Study the drawing (mm; zero at the part's minimum x, y, z) and answer. Coordinates: 2 decimals unless noted, no trailing zeros. Loops run counter-clockwise (first coordinate to the right, second up) from the corner with the lowest first, then second, coordinate; pieces in that order, holes last. Notation, with made-up numbers: (20, 15) - (47, 15) arc R8 ccw to (47, 26) - close; hole circle Ø3 at (33, 53). An arc over 180 degrees is marked (long way). Use CSV: the item, a comma, the result in double quotes.
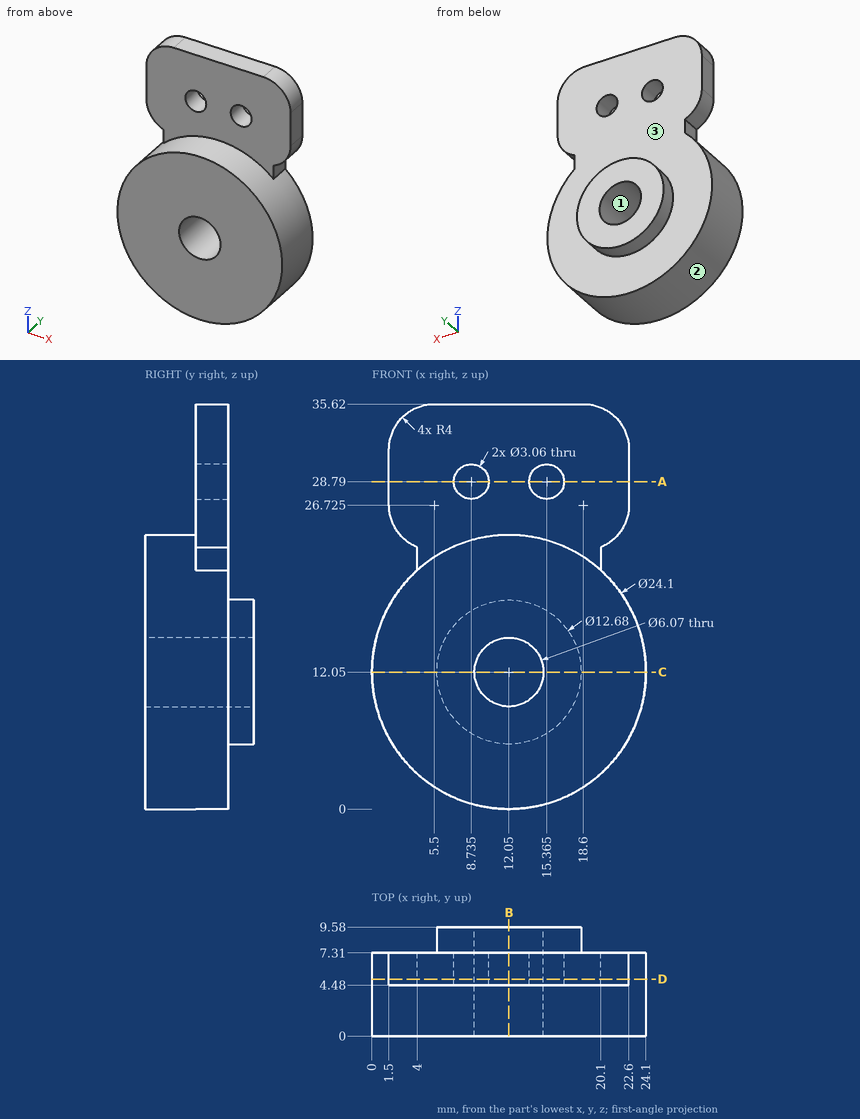
Q1. The part is cut by section A-A on z = 28.79. Determine the outline of the cut face in (x, y) (1 decimal).
Reported:
outline,"(1.5, 4.5) - (7.2, 4.5) - (7.2, 7.3) - (1.5, 7.3) - close; (10.3, 4.5) - (13.8, 4.5) - (13.8, 7.3) - (10.3, 7.3) - close; (16.9, 4.5) - (22.6, 4.5) - (22.6, 7.3) - (16.9, 7.3) - close"
Q2. Given P1, Ø0.6, axis at y = 6, z = 22, coming from the +X side; P2, Ø1, axis at y = 1.5, z = 15.5, coming from the +X side; P3, Ø8, axis at x = 5, z = 26, coming from the +Y side; P4, Ø2.5, axis at x = 8.735, z = 28.79, coming from the +Y side, each flat-ended and moving along its own axis, determine where each tip first touches the part or whether it passes through.
Reported:
P1,"stops at x = 20.1"
P2,"stops at x = 23.73"
P3,"stops at y = 7.31"
P4,"passes through"
Q3. Find the intervals of material crossed by probe 1 along X at (y, z) = (6, 28.79) (1 decimal); probe 2 along X at (y, z) = (3, 12.05) (1 decimal); probe 3 along Y at (x, z) = (8, 21.5), in increasing order. Write a range as [from, to].
Reported:
probe 1,"x = [1.5, 7.2], [10.3, 13.8], [16.9, 22.6]"
probe 2,"x = [0, 9], [15.1, 24.1]"
probe 3,"y = [0, 7.31]"
Q4. The part is cut by section B-B on x = 12.05. Determine the outline of the cut face in (y, z) (1 decimal).
Reported:
outline,"(0, 0) - (7.3, 0) - (7.3, 5.7) - (9.6, 5.7) - (9.6, 9) - (0, 9) - close; (0, 15.1) - (9.6, 15.1) - (9.6, 18.4) - (7.3, 18.4) - (7.3, 35.6) - (4.5, 35.6) - (4.5, 24.1) - (0, 24.1) - close"
Q5. The part is cut by section D-D on y = 5. Give the number of separate pieces and of enclosed holes in the cut face, and give its area (3 significant figures).
Reported:
separate pieces,"1"
enclosed holes,"3"
area,"665 mm²"
Q6. The part is cut by section C-C on z = 12.05. Determine the outline of the cut face in (x, y) (1 decimal), and give its area (3 significant figures).
Reported:
outline,"(0, 0) - (9, 0) - (9, 9.6) - (5.7, 9.6) - (5.7, 7.3) - (0, 7.3) - close; (15.1, 0) - (24.1, 0) - (24.1, 7.3) - (18.4, 7.3) - (18.4, 9.6) - (15.1, 9.6) - close"
area,"147 mm²"
Q7. For a pull along X with two mould halves and no side action, classify the marked faces 1, 2 and 3 as +X half, -X half, draft (parallel to the pull), parting line (faces both ways), or undercut.
Reported:
face 1,"undercut"
face 2,"parting line"
face 3,"draft"
